Autodesk Inventor part; units mm, degrees
ref_plane "YZ Plane" through (0, 0, 0) normal (1, 0, 0) x (0, 1, 0)
ref_plane "XZ Plane" through (0, 0, 0) normal (0, 1, 0) x (-1, 0, 0)
ref_plane "XY Plane" through (0, 0, 0) normal (0, 0, 1) x (1, 0, 0)
sketch "Sketch1" plane through (0, 0, 0) normal (0, 1, 0) x (-1, 0, 0)
  circle A0 centre (0, 0) radius 28.5
  circle A1 centre (0, 0) radius 9
  circle A2 centre (11.875, 20.5681) radius 1.5875
  circle A3 centre (-11.875, 20.5681) radius 1.5875
  circle A4 centre (23.75, 0) radius 1.5875
  circle A5 centre (11.875, -20.5681) radius 1.5875
  circle A6 centre (-11.875, -20.5681) radius 1.5875
  circle A7 centre (-23.75, 0) radius 1.5875
  dimension "d5" = 3.175
  dimension "d6" = 20.5681
  dimension "d7" = 3.175
  dimension "d8" = 3.175
  dimension "d9" = 3.175
  dimension "d10" = 3.175
  dimension "d11" = 3.175
extrude "Extrusion1" add sketch "Sketch1" along normal blind 46
sketch "Sketch2" plane through (0, 46, 0) normal (0, 1, 0) x (1, 0, 0)
  line L0 (7.5157, 0) -> (3.7578, -6.5088)
  line L1 (3.7578, -6.5088) -> (-3.7578, -6.5088)
  line L2 (-3.7578, -6.5088) -> (-7.5157, 0)
  line L3 (-7.5157, 0) -> (-3.7578, 6.5088)
  line L4 (-3.7578, 6.5088) -> (3.7578, 6.5088)
  line L5 (3.7578, 6.5088) -> (7.5157, 0)
  circle A0 centre (0, 0) radius 28.5
  circle A1 centre (-11.875, -20.5681) radius 1.5875
  circle A2 centre (11.875, -20.5681) radius 1.5875
  circle A3 centre (-23.75, 0) radius 1.5875
  circle A4 centre (-11.875, 20.5681) radius 1.5875
  circle A5 centre (23.75, 0) radius 1.5875
  circle A6 centre (11.875, 20.5681) radius 1.5875
  dimension "d4" = 13.0175
extrude "Extrusion2" add sketch "Sketch2" against normal blind 46
sketch "Sketch3" plane through (0, 46, 0) normal (0, 1, 0) x (1, 0, 0)
  circle A0 centre (-11.875, 20.5681) radius 1.5875
  circle A1 centre (-11.875, 20.5681) radius 2.3812
  circle A2 centre (11.875, 20.5681) radius 1.5875
  circle A3 centre (11.875, 20.5681) radius 2.3812
  circle A4 centre (23.75, 0) radius 1.5875
  circle A5 centre (23.75, 0) radius 2.3813
  circle A6 centre (11.875, -20.5681) radius 1.5875
  circle A7 centre (11.875, -20.5681) radius 2.3813
  circle A8 centre (-11.875, -20.5681) radius 1.5875
  circle A9 centre (-11.875, -20.5681) radius 2.3812
  circle A10 centre (-23.75, 0) radius 1.5875
  circle A11 centre (-23.75, 0) radius 2.3812
  point P0 (0, 0)
  dimension "d12" = 4.7625
  dimension "d13" = 4.7625
  dimension "d14" = 4.7625
  dimension "d15" = 4.7625
  dimension "d16" = 4.7625
  dimension "d17" = 4.7625
extrude "Extrusion3" add sketch "Sketch3" along normal blind 2.3813 and the other way blind 48.3807 contours A0 | A1 | A2 | A3 | A4 | A5 | A6 | A7 | A8 | A9 | A10 | A11
equation "\"d7\" = d5"
equation "\"d8\" = d5"
equation "\"d9\" = d5"
equation "\"d10\" = d5"
equation "\"d11\" = d5"
properties part number "new mech inside"
The listing builds one solid part. Answer for the finished solid, in the listing's coordinates (mm). A direction names the side the tool comes from. Give positions to 0.01 mm unless a question says otherwise; leave off trailing zeros. Order: outer loops, then holes, each group sorted by start corner. A loop starts at its lowest first (then second) coordinate and runs counter-clockwise, first axis right, second up. Notation, with made-up numbers: (60.25, 17) - (75.25, 17) arc R12 cw to (75.25, 33) - close; hole circle Ø9 at (42.5, 58.25). An arc over 180 degrees is marked (long way). Answer as CSV lines item,"result".
Q1. A cutting plane is placed at D-D, the plane z = 12. Determine the outline of the cut face in (x, y).
Answer key:
outline,"(-25.85, 0) - (25.85, 0) - (25.85, 46) - (-25.85, 46) - close"
Q2. A cutting plane is placed at A-A, the plane x = 0. Determine the outline of the cut face in (y, z), and give its area (3 significant figures).
Answer key:
outline,"(0, -28.5) - (46, -28.5) - (46, -6.51) - (0, -6.51) - close; (0, 6.51) - (46, 6.51) - (46, 28.5) - (0, 28.5) - close"
area,"2,020 mm^2"
Q3. A cutting plane is placed at B-B, the plane y = 22. Determine the outline of the cut face in (x, z), and give its area (4 significant figures).
Answer key:
outline,"circle Ø57 at (0, 0); hole (-7.52, 0) - (-3.76, -6.51) - (3.76, -6.51) - (7.52, 0) - (3.76, 6.51) - (-3.76, 6.51) - close"
area,"2,405 mm^2"
Q4. Each of these flat-tipped pins is pushed along its axis until it touches: pin 1 Ø1 at (x, y) = (-9.5, 37.5) entering from -Z; pin 2 Ø2.5 at (x, y) = (1.5, 13.5) entering from -Z; pin 3 Ø17 at (x, z) = (6.5, 1) entering from +Y; pin 4 Ø8 at (y, z) = (27, 4) entering from -X. Where does it stop, or does it pass through?
Answer key:
pin 1,"stops at z = -27.04"
pin 2,"stops at z = -28.5"
pin 3,"stops at y = 46"
pin 4,"stops at x = -28.5"
Q5. A cutting plane is placed at C-C, the plane x = -23.75. Determine the outline of the cut face in (y, z).
Answer key:
outline,"(-2.38, -2.38) - (0, -2.38) - (0, -15.75) - (46, -15.75) - (46, -2.38) - (48.38, -2.38) - (48.38, 2.38) - (46, 2.38) - (46, 15.75) - (0, 15.75) - (0, 2.38) - (-2.38, 2.38) - close"
Q6. Determine the mould class of faces 1 (the face through (5.663, 23.322, 3.209)), 2 (the face through (11.565, 47.207, 18.207)), 3 (the face through (12, -2.381, 21)), 4 (the face through (-26.327, 22.678, 10.916)) for opening direction X: pulls with the +X half, pulls with the -X half, needs draft (parallel to the pull), parting line crosses it, or undercut.
Answer key:
face 1,"undercut"
face 2,"undercut"
face 3,"needs draft"
face 4,"parting line crosses it"
Q7. Which of the six approach directions +Z, -Z, +X, -X, +Y, -Y give full straight-line access (tool end or side, diameter ignored) to faces 5 (the face through (12, 48.381, 21)), 6 (the face through (-12, -2.381, 21)), 7 (the face through (-5.663, 23.322, -3.209)), 8 (the face through (0, 46, 7)), 9 (the face through (0, 0, 7))?
Answer key:
face 5,"+Z, -Z, +X, -X, +Y"
face 6,"+Z, -Z, +X, -X, -Y"
face 7,"+Y, -Y"
face 8,"+Y"
face 9,"-Y"
Q8. Straight lines are drawn through the part: L1, parallel to Y at x = -13, z = 0.5; L2, parallel to X at y = 44, z = -4; L3, parallel to X at y = 5, z = 3. For each, find the intervals that lie inside material, in ascending order.
Answer key:
L1,"y = 0 to 46"
L2,"x = -28.22 to -5.21, 5.21 to 28.22"
L3,"x = -28.34 to -5.78, 5.78 to 28.34"
